Design review of the part built by this model. Coordinates are the model's own, in mm. A direction names the side the tool comes from. Give positions to 0.01 mm unless a question says otherwise; leave off trailing zeros. Loops run counter-clockwise (first coordinate to the right, second up) from the corner with the lowest first, then second, coordinate; pieces in that order, holes last. Notation, with made-up numbers: (85.5, 66) -> (113.5, 66) arc R26 ccw to (113.5, 87) -> close; hole circle Ø3 at (12.5, 19.5). An arc over 180 degrees is marked (long way). Use a Markdown table: item, result. Add a question column.
1. For pin 1 Ø3 at (y, z) = (0.5, -11) entering from -X; pin 2 Ø1 at (y, z) = (2, -9) entering from +X; pin 3 Ø1.9 at (x, z) = (-13, 2) entering from -Y; pin 4 Ø1.8 at (x, z) = (-6, -10.39) entering from +Y, all flat-tipped, find the tip position at first contact; note any pin that passes through.
2. Add section D-D (x = -2). State the section outline as (y, z) points.
3. Draft analysis for pull direction Y (two halves, no side actions). For faces 1 (the flat face through (-6.2, 2.4, -12.4)), 2 (the flat face through (-13.3, -2, 0.6)), 3 (the cylindrical face through (-14.659, 0.028, 2.887)), state which applies: pulls with the +Y half, pulls with the -Y half, needs draft (parallel to the pull), parting line crosses it, or undercut.
4. To check wall thickness, follow line 1 (X direction, y = 0.9, z = 1.4); line 2 (Y direction, x = 4.25, z = -11.25); line 3 (X direction, y = -3, z = -11.25). State the ranges of each line that lie inside material, in increasing order.
5. For faces 4 (the flat face through (-11.4, 0, 0)), 5 (the flat face through (5.9, 2.4, -12.4)), 6 (the flat face through (-13.3, 2, 0.6)), list the 3-axis set-ups (+Z, -Z, +X, -X, +Y, -Y) from which the entire face can be reached by the end or side of a thin tool; tool diameter is ignored.
6. Add section A-A (x = -6). State the section outline as (y, z) points, and give its area (3 significant figures).
7. Add section C-C (y = 1). Count the separate pieces of the cut face and the enclosed holes in it, and give its area (3 significant figures).
8. Add section B-B (y = 4). State the section outline as (x, z) points.
```python
from build123d import *

# Parameters (mm, degrees)
BOSS_EXTRUDE1_DEPTH      = 5
BOSS_EXTRUDE1_DEPTH_BACK = 5
BOSS_EXTRUDE2_DEPTH      = 2
BOSS_EXTRUDE2_DEPTH_BACK = 2
SKETCH1_3_R              = 0.5
CHAMFER1_SIZE            = 1.974397617
FILLET1_R                = 1.8
CHAMFER2_SIZE            = 0.2
BOSS_EXTRUDE3_START      = -5
BOSS_EXTRUDE3_DEPTH      = 10
CUT_EXTRUDE1_START       = -2.2
CUT_EXTRUDE1_OUTLINE_R   = 1.5
CUT_EXTRUDE1_DEPTH       = 4.6
CUT_EXTRUDE2_DEPTH       = 24.34609175
CUT_EXTRUDE2_DEPTH_BACK  = 24.34609175
SKETCH3_4_R              = 1.5
CHAMFER3_SIZE            = 0.2
CHAMFER4_SIZE            = 0.879093368


with BuildPart() as part:
    # Sketch1 → Boss-Extrude1 (new, two sides: drawn at the far end of the back side and taken through both)
    with BuildSketch(Plane(origin=(0, 0, 0), x_dir=(1, 0, 0), z_dir=(0, 1, 0)).offset(-BOSS_EXTRUDE1_DEPTH_BACK)):
        with BuildLine():
            ThreePointArc((-9.121403401, 1.2), (0, 9.2), (9.121403401, 1.2))
            Line((9.121403401, 1.2), (12.542726976, 1.2))
            ThreePointArc((12.542726976, 1.2), (11.397774814, 5.371287488), (8.909545443, 8.909545443))
            Line((8.909545443, 8.909545443), (7.963837169, 11.756585285))
            ThreePointArc((7.963837169, 11.756585285), (-6.117603026, 12.814637459), (-14.149204925, 1.2))
            Line((-14.149204925, 1.2), (-9.121403401, 1.2))
        make_face()
    extrude(amount=BOSS_EXTRUDE1_DEPTH + BOSS_EXTRUDE1_DEPTH_BACK)

    # Sketch1<3> → Boss-Extrude2 (add, two sides: drawn at the far end of the back side and taken through both)
    # profile 1 of 2: a face of its own
    with BuildSketch(Plane(origin=(0, 0, 0), x_dir=(1, 0, 0), z_dir=(0, 1, 0)).offset(-BOSS_EXTRUDE2_DEPTH_BACK)):
        Polygon((-11.4, -3.4), (-11.4, 1.2), (-14.149204925, 1.2), (-15.2, 0), (-15.2, -3.4), align=None)
        with Locations(Location((-13.2, -1.4, 0), (0, 0, 270))):
            Circle(SKETCH1_3_R, mode=Mode.SUBTRACT)
    # profile 2 of 2: a face of its own
    with BuildSketch(Plane(origin=(0, 0, 0), x_dir=(1, 0, 0), z_dir=(0, 1, 0)).offset(-BOSS_EXTRUDE2_DEPTH_BACK)):
        with BuildLine():
            ThreePointArc((9.121403401, 1.2), (9.162283589, -0.832201557), (8.755927173, -2.823781036))
            Line((8.755927173, -2.823781036), (11.11699974, -3.64230517))
            Line((11.11699974, -3.64230517), (13.6, -3.360604742))
            Line((13.6, -3.360604742), (13.6, 0))
            Line((13.6, 0), (12.542726976, 1.2))
            Line((12.542726976, 1.2), (9.121403401, 1.2))
        make_face()
        with Locations(Location((11.365493645, -1.4, 0), (0, 0, 270))):
            Circle(SKETCH1_3_R, mode=Mode.SUBTRACT)
    extrude(amount=BOSS_EXTRUDE2_DEPTH + BOSS_EXTRUDE2_DEPTH_BACK)

    # Chamfer1
    # the kernel refuses this chamfer: 1.974397617, 1.7 mm, written as the material it takes off along each edge
    with BuildSketch(Plane(origin=(-9.121403401, -10.094040977, -1.2), x_dir=(-1, 0, 0), z_dir=(0, 1, 0))) as chamfer1_piece_1:
        with BuildLine():
            Line((CHAMFER1_SIZE, 0), (-0.443747976, -1.855862617))
            ThreePointArc((-0.443747976, -1.855862617), (-0.180868647, -0.969524905), (0, 0))
            Line((0, 0), (CHAMFER1_SIZE, 0))
        make_face()
    extrude(amount=20.188081954, mode=Mode.SUBTRACT)

    # Fillet1
    fillet1_edges = [part.edges().sort_by_distance(p)[0] for p in [
        (8.755927173, 0, 2.823781036),
        (13.6, 0, 3.360604742),
        (-15.2, 0, 3.4),
        (-11.4, 0, 3.4),
    ]]
    fillet(fillet1_edges, radius=FILLET1_R)

    # Chamfer2
    chamfer2_edges = [part.edges().sort_by_distance(p)[0] for p in [
        (10.832065189, 5, -1.2),
        (-12.622502971, 5, -1.2),
    ]]
    chamfer(chamfer2_edges, length=CHAMFER2_SIZE)

    # Boss-Extrude3: read off the stored shape, not the designer's step
    # Boss-Extrude3 outline → Boss-Extrude3 (add)
    with BuildSketch(Plane(origin=(0, 0, 0), x_dir=(1, 0, 0), z_dir=(0, 1, 0)).offset(BOSS_EXTRUDE3_START)):
        with BuildLine():
            ThreePointArc((10.163659229, 7.447149191), (11.075788932, 10.888658263), (9.514234502, 14.088269654))
            ThreePointArc((9.514234502, 14.088269654), (0, 17), (-9.514234502, 14.088269654))
            ThreePointArc((-9.514234502, 14.088269654), (-10.909488785, 11.773217539), (-10.925669215, 9.070267483))
            ThreePointArc((-10.925669215, 9.070267483), (-1.999296901, 14.058549424), (7.963837169, 11.756585285))
            Line((7.963837169, 11.756585285), (8.909545443, 8.909545443))
            ThreePointArc((8.909545443, 8.909545443), (9.564592768, 8.202351199), (10.163659229, 7.447149191))
        make_face()
    extrude(amount=BOSS_EXTRUDE3_DEPTH)

    # Cut-Extrude1: read off the stored shape, not the designer's step
    # Cut-Extrude1 outline → Cut-Extrude1 (cut)
    # profile 1 of 2: a face of its own
    with BuildSketch(Plane(origin=(0, 0, 0), x_dir=(1, 0, 0), z_dir=(0, 1, 0)).offset(CUT_EXTRUDE1_START)):
        with BuildLine():
            ThreePointArc((-10.925669215, 9.070267483), (-9.629828713, 6.809799644), (-7.386560009, 5.484408011))
            ThreePointArc((-7.386560009, 5.484408011), (-4.487973836, 8.031070342), (-0.8, 9.16515139))
            Line((-0.8, 9.16515139), (-0.8, 12.76515139))
            Line((-0.8, 12.76515139), (-4.443774964, 16.408926353))
            ThreePointArc((-4.443774964, 16.408926353), (-7.074805223, 15.457914835), (-9.514234502, 14.088269654))
            ThreePointArc((-9.514234502, 14.088269654), (-10.909488785, 11.773217539), (-10.925669215, 9.070267483))
        make_face()
        with Locations((-6, 10.392304845)):
            Circle(CUT_EXTRUDE1_OUTLINE_R, mode=Mode.SUBTRACT)
    # profile 2 of 2: a face of its own
    with BuildSketch(Plane(origin=(0, 0, 0), x_dir=(1, 0, 0), z_dir=(0, 1, 0)).offset(CUT_EXTRUDE1_START)):
        with BuildLine():
            Line((0.8, 12.76515139), (0.8, 9.16515139))
            ThreePointArc((0.8, 9.16515139), (4.487973836, 8.031070342), (7.386560009, 5.484408011))
            ThreePointArc((7.386560009, 5.484408011), (8.943521978, 6.22749052), (10.163659229, 7.447149191))
            ThreePointArc((10.163659229, 7.447149191), (11.075788932, 10.888658263), (9.514234502, 14.088269654))
            ThreePointArc((9.514234502, 14.088269654), (7.074805223, 15.457914835), (4.443774964, 16.408926353))
            Line((4.443774964, 16.408926353), (0.8, 12.76515139))
        make_face()
        with Locations((6, 10.392304845)):
            Circle(CUT_EXTRUDE1_OUTLINE_R, mode=Mode.SUBTRACT)
    extrude(amount=CUT_EXTRUDE1_DEPTH, mode=Mode.SUBTRACT)

    # Sketch3<4> (on Top Plane) → Cut-Extrude2 (cut, two sides: drawn at the far end of the back side and taken through both)
    with BuildSketch(Plane(origin=(0, 0, 0), x_dir=(1, 0, 0), z_dir=(0, 1, 0)).offset(-CUT_EXTRUDE2_DEPTH_BACK)):
        with Locations(Location((-6, 10.392304845, 0), (0, 0, 270))):
            Circle(SKETCH3_4_R)
        with Locations(Location((6, 10.392304845, 0), (0, 0, 270))):
            Circle(SKETCH3_4_R)
    extrude(amount=CUT_EXTRUDE2_DEPTH + CUT_EXTRUDE2_DEPTH_BACK, mode=Mode.SUBTRACT)

    # Chamfer3
    chamfer3_edges = [part.edges().sort_by_distance(p)[0] for p in [
        (10.832065189, -5, -1.2),
        (-12.622502971, -5, -1.2),
    ]]
    chamfer(chamfer3_edges, length=CHAMFER3_SIZE)

    # Chamfer4
    # the kernel refuses this chamfer: 1.2, 0.879093368, 0.860893535 mm, written as the material it takes off along each edge
    with BuildSketch(Plane(origin=(-10.925669215, -2.2, -9.070267483), x_dir=(0.39004090041873263, 0, 0.9207975325773544), z_dir=(0, 1, 0))) as chamfer4_piece_1:
        with BuildLine():
            Line((1.40776743, 0), (0.416367157, -0.748890719))
            ThreePointArc((0.416367157, -0.748890719), (0.204153797, -0.380499927), (0, 0))
            ThreePointArc((0, 0), (0.723274519, -0.048770435), (1.40776743, 0))
        make_face()
    extrude(amount=4.6, mode=Mode.SUBTRACT)
    with BuildSketch(Plane(origin=(4.443774964, -2.2, -16.408926353), x_dir=(-0.9735942522545705, 0, -0.22828541779286665), z_dir=(0, 1, 0))) as chamfer4_piece_2:
        with BuildLine():
            Line((1.16103032, 0), (CHAMFER4_SIZE * 0.527012931132, CHAMFER4_SIZE * 0.849857264932))
            Line((CHAMFER4_SIZE * 0.527012931132, CHAMFER4_SIZE * 0.849857264932), (0, 0))
            ThreePointArc((0, 0), (0.596888963, -0.009906707), (1.16103032, 0))
        make_face()
    extrude(amount=4.6, mode=Mode.SUBTRACT)
    with BuildSketch(Plane(origin=(-4.443774964, -2.2, -16.408926353), x_dir=(0.9735942522545713, 0, -0.22828541779286343), z_dir=(0, 1, 0))) as chamfer4_piece_3:
        with BuildLine():
            Line((1.16103032, 0), (CHAMFER4_SIZE * 0.527012931132, -CHAMFER4_SIZE * 0.849857264932))
            Line((CHAMFER4_SIZE * 0.527012931132, -CHAMFER4_SIZE * 0.849857264932), (0, 0))
            ThreePointArc((0, 0), (0.596888963, 0.009906707), (1.16103032, 0))
        make_face()
    extrude(amount=4.6, mode=Mode.SUBTRACT)


solid = part.part
```
Taken from the geometry:
| question | item | result |
|---|---|---|
| 1 | pin 1 | stops at x = -0.8 |
| 1 | pin 2 | stops at x = 10.98 |
| 1 | pin 3 | stops at y = -2 |
| 1 | pin 4 | passes through |
| 2 | outline | (-5, -16.88) -> (5, -16.88) -> (5, -8.98) -> (2.4, -8.98) -> (2.4, -13.97) -> (-2.2, -13.97) -> (-2.2, -8.98) -> (-5, -8.98) -> close |
| 3 | face 1 | undercut |
| 3 | face 2 | pulls with the -Y half |
| 3 | face 3 | needs draft |
| 4 | line 1 | x = -15.2 to -13.7, -12.7 to -11.4, 9.09 to 10.87, 11.87 to 13.6 |
| 4 | line 2 | y = -5 to -2.2, 2.4 to 5 |
| 4 | line 3 | x = -11.03 to -7.23, -4.77 to 4.77, 7.23 to 11.03 |
| 5 | face 4 | +Z, +Y, -Y |
| 5 | face 5 | none |
| 5 | face 6 | +Z, +X, -X, +Y |
| 6 | outline | (-5, -15.91) -> (-2.2, -15.91) -> (-2.2, -11.89) -> (-5, -11.89) -> close; (-5, -8.89) -> (-2.2, -8.89) -> (-2.2, -6.97) -> (-5, -6.97) -> close; (2.4, -15.91) -> (5, -15.91) -> (5, -11.89) -> (2.4, -11.89) -> close; (2.4, -8.89) -> (5, -8.89) -> (5, -6.97) -> (2.4, -6.97) -> close |
| 6 | area | 32.0 mm^2 |
| 7 | separate pieces | 3 |
| 7 | enclosed holes | 2 |
| 7 | area | 108 mm^2 |
| 8 | outline | (-14.15, -1.2) arc R14.2 ccw to (-10.93, -9.07) arc R5.1 ccw to (-9.51, -14.09) arc R17 ccw to (9.51, -14.09) arc R5.1 ccw to (10.16, -7.45) arc R12.6 ccw to (12.54, -1.2) -> (9.12, -1.2) arc R9.2 cw to (-8.68, -3.06) -> (-11.1, -1.2) -> close; hole circle Ø3 at (-6, -10.39); hole circle Ø3 at (6, -10.39) |
